Build history of the part. All positions in model axes, mm. Face numbers are marked on the shaded views. A direction names the side the tool comes from. Round coordinates to 2 decimals unless told otherwise and drop trailing zeros. Write each loop counter-clockwise with the first axis right and the second up, starting at its lowest first coordinate (ties: lowest second). Pieces come first, ordered by that corner, then holes.
from build123d import *

# Parameters (mm, degrees)
BOX006_W          = 5
BOX006_H          = 5
BOX006_DEPTH      = 3.9
CYLINDER003_R     = 2
CYLINDER003_DEPTH = 10
CYLINDER002_R     = 6.25
CYLINDER002_DEPTH = 10
BOX004_W          = 10
BOX004_H          = 5
BOX004_DEPTH      = 4.5
BOX003_W          = 20
BOX003_H          = 10
BOX003_DEPTH      = 10
CYLINDER001_R     = 6.25
CYLINDER001_DEPTH = 5
CYLINDER_R        = 7.25
CYLINDER_DEPTH    = 5
BOX_W             = 24
BOX_H             = 25
BOX_DEPTH         = 3
BOX001_W          = 1.5
BOX001_H          = 4.5
BOX001_DEPTH      = 5
BOX002_W          = 2.5
BOX002_H          = 4.5
BOX002_DEPTH      = 1.5
BOX005_W          = 13
BOX005_H          = 1
BOX005_DEPTH      = 5.5
BOX007_W          = 12.5
BOX007_H          = 1
BOX007_DEPTH      = 2.75


with BuildPart() as cube006:
    # Box006 → Box006 (new body)
    with BuildSketch(Plane(origin=(10, 8, -3.9), x_dir=(1, 0, 0), z_dir=(0, 0, 1))):
        with Locations((2.5, 2.5)):
            Rectangle(BOX006_W, BOX006_H)
    extrude(amount=BOX006_DEPTH)


with BuildPart() as cylinder003:
    # Cylinder003 → Cylinder003 (new body)
    with BuildSketch(Plane(origin=(12.5, 18.5, 0), x_dir=(1, 0, 0), z_dir=(0, 0, 1))):
        Circle(CYLINDER003_R)
    extrude(amount=CYLINDER003_DEPTH)


with BuildPart() as cylinder002:
    # Cylinder002 → Cylinder002 (new body)
    with BuildSketch(Plane(origin=(14.5, 30, -7), x_dir=(1, 0, 0), z_dir=(0, -1, 0))):
        Circle(CYLINDER002_R)
    extrude(amount=CYLINDER002_DEPTH)


with BuildPart() as cut004:
    # Box004 → Box004 (new body)
    with BuildSketch(Plane(origin=(9.5, 25, -1.5), x_dir=(1, 0, 0), z_dir=(0, 0, 1))):
        with Locations((5, 2.5)):
            Rectangle(BOX004_W, BOX004_H)
    extrude(amount=BOX004_DEPTH)

    # Cut004: cut Cylinder002
    add(cylinder002.part, mode=Mode.SUBTRACT)


with BuildPart() as cube003:
    # Box003 → Box003 (new body)
    with BuildSketch(Plane(origin=(5, 25, -17), x_dir=(1, 0, 0), z_dir=(0, 0, 1))):
        with Locations((10, 5)):
            Rectangle(BOX003_W, BOX003_H)
    extrude(amount=BOX003_DEPTH)


with BuildPart() as cylinder001:
    # Cylinder001 → Cylinder001 (new body)
    with BuildSketch(Plane(origin=(14.5, 30, -4.5), x_dir=(1, 0, 0), z_dir=(0, -1, 0))):
        Circle(CYLINDER001_R)
    extrude(amount=CYLINDER001_DEPTH)


with BuildPart() as fusion002:
    # Cylinder → Cylinder (new body)
    with BuildSketch(Plane(origin=(14.5, 30, -4.5), x_dir=(1, 0, 0), z_dir=(0, -1, 0))):
        Circle(CYLINDER_R)
    extrude(amount=CYLINDER_DEPTH)

    # Cut002: cut Cylinder001
    add(cylinder001.part, mode=Mode.SUBTRACT)


with BuildPart() as fusion002_1:
    # Cut002 placement: moved
    add(fusion002.part.moved(Location((0, 0, -2.5))))

    # Cut003: cut Cube003
    add(cube003.part, mode=Mode.SUBTRACT)

    # Fusion002: union Cut004
    add(cut004.part)


with BuildPart() as cone001:
    # Cone001 → Cone001 (revolve)
    with BuildSketch(Plane(origin=(3, 21, 0), x_dir=(1, 0, 0), z_dir=(0, -1, 0))):
        Polygon((0, 0), (1.25, 0), (2.75, 3), (0, 3), align=None)
    revolve(axis=Axis((3, 21, 0), (0, 0, 1)))


with BuildPart() as cone:
    # Cone → Cone (revolve)
    with BuildSketch(Plane(origin=(3, 4, 0), x_dir=(1, 0, 0), z_dir=(0, -1, 0))):
        Polygon((0, 0), (1.25, 0), (2.75, 3), (0, 3), align=None)
    revolve(axis=Axis((3, 4, 0), (0, 0, 1)))


with BuildPart() as cut001:
    # Box → Box (new body)
    with BuildSketch(Plane.XY):
        with Locations((12, 12.5)):
            Rectangle(BOX_W, BOX_H)
    extrude(amount=BOX_DEPTH)

    # Cut: cut Cone
    add(cone.part, mode=Mode.SUBTRACT)

    # Cut001: cut Cone001
    add(cone001.part, mode=Mode.SUBTRACT)


with BuildPart() as cube001:
    # Box001 → Box001 (new body)
    with BuildSketch(Plane(origin=(21.5, 4.75, -3.5), x_dir=(1, 0, 0), z_dir=(0, 0, 1))):
        with Locations((0.75, 2.25)):
            Rectangle(BOX001_W, BOX001_H)
    extrude(amount=BOX001_DEPTH)


with BuildPart() as fusion003:
    # Box002 → Box002 (new body)
    with BuildSketch(Plane(origin=(21.5, 4.75, -3.5), x_dir=(1, 0, 0), z_dir=(0, 0, 1))):
        with Locations((1.25, 2.25)):
            Rectangle(BOX002_W, BOX002_H)
    extrude(amount=BOX002_DEPTH)

    # Fusion: union Cube001
    add(cube001.part)

    # Fusion001: union Cut001
    add(cut001.part)

    # Fusion003: union Fusion002
    add(fusion002_1.part)


with BuildPart() as fusion005:
    # Box005 → Box005 (new body)
    with BuildSketch(Plane(origin=(8, 24, -5.5), x_dir=(1, 0, 0), z_dir=(0, 0, 1))):
        with Locations((6.5, 0.5)):
            Rectangle(BOX005_W, BOX005_H)
    extrude(amount=BOX005_DEPTH)

    # Fusion004: union Fusion003
    add(fusion003.part)

    # Cut005: cut Cylinder003
    add(cylinder003.part, mode=Mode.SUBTRACT)

    # Fusion005: union Cube006
    add(cube006.part)


with BuildPart() as fusion006:
    # Box007 → Box007 (new body)
    with BuildSketch(Plane(origin=(8.25, 0, -2.75), x_dir=(1, 0, 0), z_dir=(0, 0, 1))):
        with Locations((6.25, 0.5)):
            Rectangle(BOX007_W, BOX007_H)
    extrude(amount=BOX007_DEPTH)

    # Fusion006: union Fusion005
    add(fusion005.part)


solid = fusion006.part
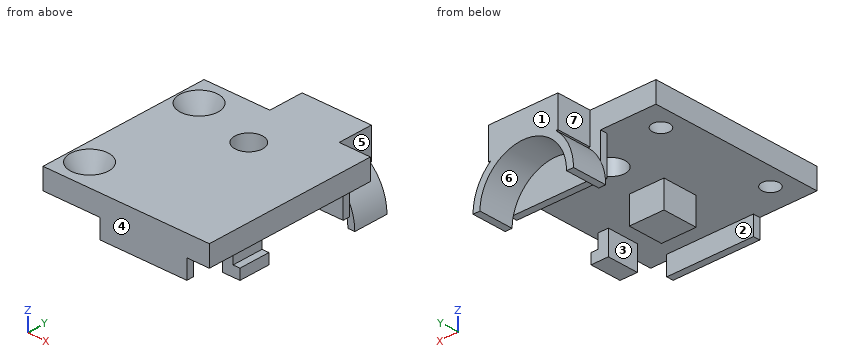
1) Wall check: L1, parallel to X at y = 18.5, z = 1.8; L2, parallel to Y at x = 12.5, z = 0.85; L3, parallel to Y at x = 18.5, z = -2.25. Give the ranges that are in metal, low to high.
Results:
L1: x = 0 to 10.5, 14.5 to 24
L2: y = 0 to 16.5, 20.5 to 30
L3: y = 0 to 1, 24 to 25
2) Slice it at C-C (x = 11.25). Write the cut outline in (y, z).
Results:
outline: (0, -2.75) - (1, -2.75) - (1, 0) - (8, 0) - (8, -3.9) - (13, -3.9) - (13, 0) - (16.94, 0) - (16.94, 3) - (0, 3) - close; (20.06, 0) - (24, 0) - (24, -5.5) - (25, -5.5) - (25, -1.66) - (30, -1.66) - (30, 3) - (20.06, 3) - close
3) Slice it at D-D (y = 28.25). Write the cut outline in (x, z), plus the area to 3 significant figures.
Results:
outline: (7.25, -7) - (8.25, -7) arc R6.25 cw to (20.75, -7) - (21.75, -7) arc R7.25 ccw to (19.22, -1.5) - (19.5, -1.5) - (19.5, 3) - (9.5, 3) - (9.5, -1.5) - (9.78, -1.5) arc R7.25 ccw to start
area: 54.9 mm2
4) Which spindle directions (+Z, -Z, +X, -X, +Y, -Y) get a long thin tool onto all of the face, cutting with end or side? Do the marked faces 5, 6 and 7. Say none if no direction does.
Results:
face 5: +Z, +X, +Y
face 6: -Z, +Y
face 7: +Z, -X, +Y
5) Mould opens along Y. For the marked faces 1, 2, 3 and 4 say: released by +Y, released by -Y, zero draft, split by the parting line, or undercut.
Results:
face 1: released by +Y
face 2: undercut
face 3: zero draft
face 4: released by -Y
6) Slice it at A-A (y = 21). Write the cut outline in (x, z).
Results:
outline: (0, 0) - (1.75, 0) - (0.25, 3) - (0, 3) - close; (4.25, 0) - (24, 0) - (24, 3) - (5.75, 3) - close
7) Slice it at B-B (x = 3). Write the cut outline in (y, z).
Results:
outline: (0, 0) - (2.75, 0) - (1.25, 3) - (0, 3) - close; (5.25, 0) - (19.75, 0) - (18.25, 3) - (6.75, 3) - close; (22.25, 0) - (25, 0) - (25, 3) - (23.75, 3) - close
8) Pin check, flat tips, straight feed: pin 1 Ø5 at (y, z) = (28.5, 1) entering from +X; pin 2 Ø2 at (x, z) = (5.5, 0.5) entering from +Y; pin 3 Ø2 at (x, y) = (22.5, 6.5) entering from -Z. Stop position of each tip, or through.
Results:
pin 1: stops at x = 19.5
pin 2: stops at y = 25
pin 3: stops at z = -3.5
